```python
from build123d import *

# Parameters (mm, degrees)
BLANKSKE_W         = 17
BLANKSKE_H         = 3.3
BLANK_DEPTH        = 2
TOOTHCUTSIM_DEPTH  = 18.432441022
TEETHCUTS_COUNT    = 19
TEETHCUTS_PITCH    = 0.942477795
SKETCH1_W          = 0.5
SKETCH1_H          = 0.5
CUT_EXTRUDE1_DEPTH = 18.432441022


with BuildPart() as part:
    # BlankSke → Blank (new body)
    with BuildSketch(Plane.XY):
        with Locations((8.5, 1.65)):
            Rectangle(BLANKSKE_W, BLANKSKE_H)
    extrude(amount=-BLANK_DEPTH)

    # TooCutSkeSim → ToothCutSim (cut, through all)
    with BuildSketch(Plane.XY):
        Polygon((0.129130611, 2.625), (-0.129130611, 2.625), (-0.384055363, 3.3254), (0.384055363, 3.3254), align=None)
    toothcutsim = extrude(amount=-TOOTHCUTSIM_DEPTH, mode=Mode.SUBTRACT)

    # TeethCuts: ToothCutSim ×19
    with Locations(*[(i * TEETHCUTS_PITCH, 0, 0) for i in range(1, TEETHCUTS_COUNT)]):
        add(toothcutsim, mode=Mode.SUBTRACT)

    # Sketch1 → Cut-Extrude1 (cut, through all)
    with BuildSketch(Plane(origin=(17, 0, 0), x_dir=(0, 0, -1), z_dir=(1, 0, 0))):
        with Locations((1, 0.25)):
            Rectangle(SKETCH1_W, SKETCH1_H)
    extrude(amount=-CUT_EXTRUDE1_DEPTH, mode=Mode.SUBTRACT)

    # Loft1: read off the stored shape, not the designer's step
    # Loft1: loft between two sections, ruled curve by curve
    loft1_from = [
        Edge.make_bspline([(-1, 2.321360982, -1.672573988), (-1, 2.386469579, -1.574911092), (-1, 2.485564206, -1.365149558), (-1, 2.540372571, -1.027786651), (-1, 2.500881486, -0.688289756), (-1, 2.411377214, -0.474260245), (-1, 2.350753212, -0.373752031)], [0, 0, 0, 0, 0.25, 0.5, 0.75, 1, 1, 1, 1], 3),
        Edge.make_bspline([(-1, 2.350753212, -0.373752031), (-1, 2.25171936, -0.20956433), (-1, 1.98438986, 0.062051662), (-1, 1.433501665, 0.252036945), (-1, 0.856426864, 0.171062344), (-1, 0.542030673, -0.044333441), (-1, 0.413387868, -0.186517595)], [0, 0, 0, 0, 0.25, 0.5, 0.75, 1, 1, 1, 1], 3),
        Edge.make_bspline([(-1, 0.455133028, -1.857366972), (-1, 0.583554487, -1.985788432), (-1, 0.889022109, -2.17852057), (-1, 1.435989481, -2.247122683), (-1, 1.958881136, -2.07258365), (-1, 2.220618901, -1.82368711), (-1, 2.321360982, -1.672573988)], [0, 0, 0, 0, 0.25, 0.5, 0.75, 1, 1, 1, 1], 3),
        Edge.make_bspline([(-1, 0.413387868, -0.186517595), (-1, 0.375553122, -0.228334946), (-1, 0.306844772, -0.315959172), (-1, 0.223712602, -0.45807693), (-1, 0.160449665, -0.610084219), (-1, 0.131966282, -0.717729651), (-1, 0.103213139, -0.868683652), (-1, 0.089654768, -1.065841054), (-1, 0.141987611, -1.360301974), (-1, 0.264270675, -1.633156172), (-1, 0.386349144, -1.788583089), (-1, 0.455133028, -1.857366972)], [0, 0, 0, 0, 0.0917447, 0.183489399, 0.275234099, 0.366978799, 0.366978799, 0.525234099, 0.683489399, 0.8417447, 1, 1, 1, 1], 3),
    ]
    loft1_to = [
        Edge.make_bspline([(0, 2.625, -2), (0, 2.625, -1.833333333), (0, 2.625, -1.5), (0, 2.625, -1), (0, 2.625, -0.5), (0, 2.625, -0.166666667), (0, 2.625, 0)], [0, 0, 0, 0, 0.25, 0.5, 0.75, 1, 1, 1, 1], 3),
        Edge.make_bspline([(0, 2.625, 0), (0, 2.40625, 0), (0, 1.96875, 0), (0, 1.3125, 0), (0, 0.65625, 0), (0, 0.21875, 0), (0, 0, 0)], [0, 0, 0, 0, 0.25, 0.5, 0.75, 1, 1, 1, 1], 3),
        Edge.make_bspline([(0, 0, -2), (0, 0.21875, -2), (0, 0.65625, -2), (0, 1.3125, -2), (0, 1.96875, -2), (0, 2.40625, -2), (0, 2.625, -2)], [0, 0, 0, 0, 0.25, 0.5, 0.75, 1, 1, 1, 1], 3),
        Edge.make_bspline([(0, 0, 0), (0, 0, -0.061163133), (0, 0, -0.185429777), (0, 0, -0.375), (0, 0, -0.564570223), (0, 0, -0.688836867), (0, 0, -0.855503534), (0, 0, -1.064467717), (0, 0, -1.375), (0, 0, -1.685532283), (0, 0, -1.894496466), (0, 0, -2)], [0, 0, 0, 0, 0.0917447, 0.183489399, 0.275234099, 0.366978799, 0.366978799, 0.525234099, 0.683489399, 0.8417447, 1, 1, 1, 1], 3),
    ]
    loft1 = Solid(Shell([*[Face.make_surface_from_curves(loft1_from[k], loft1_to[k]) for k in range(4)], Face(Wire(loft1_from)), Face(Wire(loft1_to))]))
    add(loft1)


solid = part.part
```
The listing builds one solid part. Answer for the finished solid, in the listing's coordinates (mm). A direction names the side the tool comes from. Round coordinates to 2 decimals unless told otherwise and drop trailing zeros.
Q1. Given pin 1 Ø1 at (x, y) = (14, 2.5) entering from +Z, flat-ended and moving along its own axis, determine where the tip first touches the part or whether it passes through.
Q2. Find the intervals of material crossed by line 1 (Y direction, x = 13.25, z = -0.5) (3 decimals); line 2 (Z direction, x = 11.25, y = 1.8); line 3 (Y direction, x = 12.25, z = -0.95) (3 decimals), in increasing order.
Q3. Which of the six approach directions +Z, -Z, +X, -X, +Y, -Y give full straight-line access (tool end or side, diameter ignored) to faces 1 (the face through (8, 1, 0)), 2 (the face through (17, 1, -1)), 3 (the face through (8, 1, -2))?
Completed:
1. pin 1: stops at z = 0
2. line 1: y = 0 to 2.625
2. line 2: z = -2 to 0
2. line 3: y = 0.5 to 2.625
3. face 1: +Z, +X, +Y, -Y
3. face 2: +Z, -Z, +X, +Y, -Y
3. face 3: -Z, +X, +Y, -Y
